Work out the finished part from the listing and answer in its coordinate system (mm). A direction names the side the tool comes from. Round coordinates to 2 decimals unless told otherwise and drop trailing zeros. Write each loop counter-clockwise with the first axis right and the second up, starting at its lowest first coordinate (ties: lowest second). Pieces come first, ordered by that corner, then holes. Notation, with made-up numbers: (-39, 41) -> (3, 41) arc R12 cw to (3, 50) -> close; hole circle Ø11 at (57.5, 10.25). An arc over 180 degrees is marked (long way). Answer as a JSON object with one key per item and string values. Group by question number.
from build123d import *

# Parameters (mm, degrees)
F3_DEPTH = 22.353
F4_D     = 2.2606
F4_DEPTH = 9.652
F4_TIP   = 0.6791527577


with BuildPart() as f1:
    # F0 (on Front) → F1 (revolve)
    with BuildSketch(Plane.XZ):
        Polygon((-18.8786415076, 13.7577650476), (-41.2306415076, 10.6163963103), (-41.2306415076, 3.5297963103), (-18.8786415076, 3.5297963103), align=None)
    revolve(axis=Axis((-30.0546415076, 0, -2.8202036897), (1, 0, 0)))

    # F2 (on face) → F3 (cut, through all)
    with BuildSketch(Plane(origin=(-41.2306415076, 0, 0), x_dir=(0, -1, 0), z_dir=(-1, 0, 0))):
        with BuildLine():
            Line((13.4341990293, -2.5662036897), (6.3449179664, -2.5662036897))
            ThreePointArc((6.3449179664, -2.5662036897), (6.3487293645, -2.6931782719), (6.35, -2.8202036897))
            ThreePointArc((6.35, -2.8202036897), (6.3487293645, -2.9472291075), (6.3449179664, -3.0742036897))
            Line((6.3449179664, -3.0742036897), (13.4341990293, -3.0742036897))
            ThreePointArc((13.4341990293, -3.0742036897), (13.4359997439, -2.9472093634), (13.4366, -2.8202036897))
            ThreePointArc((13.4366, -2.8202036897), (13.4359997439, -2.6931980159), (13.4341990293, -2.5662036897))
        make_face()
        with BuildLine():
            Line((16.5760227876, -2.5662036897), (13.4341990293, -2.5662036897))
            ThreePointArc((13.4341990293, -2.5662036897), (13.4359997439, -2.6931980159), (13.4366, -2.8202036897))
            ThreePointArc((13.4366, -2.8202036897), (13.4359997439, -2.9472093634), (13.4341990293, -3.0742036897))
            Line((13.4341990293, -3.0742036897), (16.5760227876, -3.0742036897))
            ThreePointArc((16.5760227876, -3.0742036897), (16.5774822427, -2.9472074167), (16.5779687373, -2.8202036897))
            ThreePointArc((16.5779687373, -2.8202036897), (16.5774822427, -2.6931999627), (16.5760227876, -2.5662036897))
        make_face()
    extrude(amount=-F3_DEPTH, mode=Mode.SUBTRACT)

    # F4
    with Locations(Plane(origin=(-41.2306415076, 0, 0), x_dir=(0, -1, 0), z_dir=(-1, 0, 0))):
        with Locations((-7.7230202641, 4.9028165744), (7.7230202641, 4.9028165744), (7.7230202641, -10.5432239538), (-7.7230202641, -10.5432239538)):
            Hole(F4_D / 2, depth=F4_DEPTH)
            with Locations((0, 0, -(F4_DEPTH + F4_TIP / 2))):  # 118° drill point
                Cone(0, F4_D / 2, F4_TIP, mode=Mode.SUBTRACT)


solid = f1.part
1) A cutting plane is placed at A-A on x = -27. Determine the outline of the cut face in (y, z), plus the area to 3 significant figures.
2) Straight lines are drawn through the part: L1, parallel to Z at x = -32.5, y = -2; L2, parallel to Z at x = -30, y = 3.5; L3, parallel to Y at x = -39.25, z = -4.5. For each, find the intervals that lie inside material, in ascending order.
3) A tool of negligible diameter and unlimited length cuts with its end or side. For faces 1 (the face through (-30, -10, -2.566)), 2 (the face through (-41.231, 6, 0)), 3 (the face through (-36.34, -7.12, 5.86)), from which of +Z, -Z, +X, -X, +Y, -Y can it reach the whole face along a straight path? Write none if from no direction.
4) Each of these flat-tipped pins is pushed along its axis until it touches: P1, Ø2, axis at x = -25, z = 5, coming from the -Y side; P2, Ø2, axis at x = -21.5, z = -12, coming from the +Y side; P3, Ø10, axis at y = 0, z = -2.82, coming from the +X side; P4, Ø5, axis at x = -30, y = -13.5, coming from the -Z side. Where does it stop, or does it pass through?
5) A cutting plane is placed at B-B on x = -24.25. Determine the outline of the cut face in (y, z), plus the area to 3 significant figures.
6) For a pull along Z with two mould halves and no side action, classify faces 4 (the face through (-31.017, -7.697, -10.349)), 5 (the face through (-18.879, 7, -3)) as released by +Z, released by -Z, zero draft, split by the parting line, or undercut.
Established:
{
 "1": {"outline": "(-15.43, -3.07) arc R15.44 ccw (long way) to (-15.43, -2.57) -> (-6.34, -2.57) arc R6.35 cw (long way) to (-6.34, -3.07) -> close", "area": "617 mm²"},
 "2": {"L1": "z = -17.35 to -8.85, 3.21 to 11.71", "L2": "z = -17.42 to -8.12, 2.48 to 11.78", "L3": "y = -13.61 to -6.12, 6.12 to 13.61"},
 "3": {"face 1": "+X, -X, -Y", "face 2": "+Z, -Z, -X, +Y, -Y", "face 3": "-X"},
 "4": {"P1": "stops at y = -14.19", "P2": "stops at y = 14.02", "P3": "passes through", "P4": "stops at z = -13.09"},
 "5": {"outline": "(-15.82, -3.07) arc R15.82 ccw (long way) to (-15.82, -2.57) -> (-6.34, -2.57) arc R6.35 cw (long way) to (-6.34, -3.07) -> close", "area": "655 mm²"},
 "6": {"face 4": "undercut", "face 5": "zero draft"}
}
